Autodesk Inventor part; units mm, degrees
ref_plane "ip_cb_11_1_XY" through (2.3526, 9.0717, 3.7576) normal (1, 0, 0) x (0, 0, -1)
ref_plane "ip_cb_11_1_YZ" through (2.3526, 9.0717, 3.7576) normal (0, 0, -1) x (0, 1, 0)
ref_plane "ip_cb_11_1_ZX" through (2.3526, 9.0717, 3.7576) normal (0, 1, 0) x (1, 0, 0)
sketch "Sketch_1" plane through (0, 0, 0) normal (0, 0, 1) x (1, 0, 0)
  line L0 (14, 0) -> (0, 0)
  arc A0 (0, 5.6) -> (0.6, 5) centre (0.6, 5.6) ccw
  line L1 (0.6, 5) -> (13.4, 5)
  arc A1 (13.4, 5) -> (14, 5.6) centre (13.4, 5.6) ccw
  line L2 (14, 5.6) -> (14, 7.6)
  line L3 (14, 7.6) -> (12.4286, 7.6)
  arc A2 (10.8662, 7.6) -> (12.4286, 7.6) centre (11.6474, 9.8192) ccw
  line L4 (10.8662, 7.6) -> (3.1338, 7.6)
  arc A3 (1.5714, 7.6) -> (3.1338, 7.6) centre (2.3526, 9.8192) ccw
  line L5 (1.5714, 7.6) -> (0, 7.6)
  line L6 (0, 7.6) -> (0, 5.6)
revolve "Revolution1" add sketch "Sketch_1" angle 360 about axis through (14, 0, 0) along (1, 0, 0)
ref_plane "ip_cb_11_1_XY" through (2.3526, 9.0717, 3.7576) normal (1, 0, 0) x (0, 0, -1)
ref_plane "ip_cb_11_1_YZ" through (2.3526, 9.0717, 3.7576) normal (0, 0, -1) x (0, 1, 0)
ref_plane "ip_cb_11_1_ZX" through (2.3526, 9.0717, 3.7576) normal (0, 1, 0) x (1, 0, 0)
ref_plane "ip_cb_11_2_XY" through (2.3526, 3.7576, 9.0717) normal (1, 0, 0) x (0, 0, -1)
ref_plane "ip_cb_11_2_YZ" through (2.3526, 3.7576, 9.0717) normal (0, 0, -1) x (0, 1, 0)
ref_plane "ip_cb_11_2_ZX" through (2.3526, 3.7576, 9.0717) normal (0, 1, 0) x (1, 0, 0)
ref_plane "ip_cb_11_3_XY" through (2.3526, -3.7576, 9.0717) normal (1, 0, 0) x (0, 0, -1)
ref_plane "ip_cb_11_3_YZ" through (2.3526, -3.7576, 9.0717) normal (0, 0, -1) x (0, 1, 0)
ref_plane "ip_cb_11_3_ZX" through (2.3526, -3.7576, 9.0717) normal (0, 1, 0) x (1, 0, 0)
ref_plane "ip_cb_11_4_XY" through (2.3526, -9.0717, 3.7576) normal (1, 0, 0) x (0, 0, -1)
ref_plane "ip_cb_11_4_YZ" through (2.3526, -9.0717, 3.7576) normal (0, 0, -1) x (0, 1, 0)
ref_plane "ip_cb_11_4_ZX" through (2.3526, -9.0717, 3.7576) normal (0, 1, 0) x (1, 0, 0)
ref_plane "ip_cb_11_5_XY" through (2.3526, -9.0717, -3.7576) normal (1, 0, 0) x (0, 0, -1)
ref_plane "ip_cb_11_5_YZ" through (2.3526, -9.0717, -3.7576) normal (0, 0, -1) x (0, 1, 0)
ref_plane "ip_cb_11_5_ZX" through (2.3526, -9.0717, -3.7576) normal (0, 1, 0) x (1, 0, 0)
ref_plane "ip_cb_11_6_XY" through (2.3526, -3.7576, -9.0717) normal (1, 0, 0) x (0, 0, -1)
ref_plane "ip_cb_11_6_YZ" through (2.3526, -3.7576, -9.0717) normal (0, 0, -1) x (0, 1, 0)
ref_plane "ip_cb_11_6_ZX" through (2.3526, -3.7576, -9.0717) normal (0, 1, 0) x (1, 0, 0)
ref_plane "ip_cb_11_7_XY" through (2.3526, 3.7576, -9.0717) normal (1, 0, 0) x (0, 0, -1)
ref_plane "ip_cb_11_7_YZ" through (2.3526, 3.7576, -9.0717) normal (0, 0, -1) x (0, 1, 0)
ref_plane "ip_cb_11_7_ZX" through (2.3526, 3.7576, -9.0717) normal (0, 1, 0) x (1, 0, 0)
ref_plane "ip_cb_11_8_XY" through (2.3526, 9.0717, -3.7576) normal (1, 0, 0) x (0, 0, -1)
ref_plane "ip_cb_11_8_YZ" through (2.3526, 9.0717, -3.7576) normal (0, 0, -1) x (0, 1, 0)
ref_plane "ip_cb_11_8_ZX" through (2.3526, 9.0717, -3.7576) normal (0, 1, 0) x (1, 0, 0)
ref_plane "ip_cb_1a_XY" through (0, 0, 0) normal (-1, 0, 0) x (0, 0, -1)
ref_plane "ip_cb_1a_YZ" through (0, 0, 0) normal (0, 0, -1) x (0, -1, 0)
ref_plane "ip_cb_1a_ZX" through (0, 0, 0) normal (0, -1, 0) x (-1, 0, 0)
ref_plane "ip_cb_22_1_XY" through (11.6474, 9.8192, 0) normal (1, 0, 0) x (0, 0, -1)
ref_plane "ip_cb_22_1_YZ" through (11.6474, 9.8192, 0) normal (0, 0, -1) x (0, 1, 0)
ref_plane "ip_cb_22_1_ZX" through (11.6474, 9.8192, 0) normal (0, 1, 0) x (1, 0, 0)
ref_plane "ip_cb_22_2_XY" through (11.6474, 6.9432, 6.9432) normal (1, 0, 0) x (0, 0, -1)
ref_plane "ip_cb_22_2_YZ" through (11.6474, 6.9432, 6.9432) normal (0, 0, -1) x (0, 1, 0)
ref_plane "ip_cb_22_2_ZX" through (11.6474, 6.9432, 6.9432) normal (0, 1, 0) x (1, 0, 0)
ref_plane "ip_cb_22_3_XY" through (11.6474, 0, 9.8192) normal (1, 0, 0) x (0, 0, -1)
ref_plane "ip_cb_22_3_YZ" through (11.6474, 0, 9.8192) normal (0, 0, -1) x (0, 1, 0)
ref_plane "ip_cb_22_3_ZX" through (11.6474, 0, 9.8192) normal (0, 1, 0) x (1, 0, 0)
ref_plane "ip_cb_22_4_XY" through (11.6474, -6.9432, 6.9432) normal (1, 0, 0) x (0, 0, -1)
ref_plane "ip_cb_22_4_YZ" through (11.6474, -6.9432, 6.9432) normal (0, 0, -1) x (0, 1, 0)
ref_plane "ip_cb_22_4_ZX" through (11.6474, -6.9432, 6.9432) normal (0, 1, 0) x (1, 0, 0)
ref_plane "ip_cb_22_5_XY" through (11.6474, -9.8192, 0) normal (1, 0, 0) x (0, 0, -1)
ref_plane "ip_cb_22_5_YZ" through (11.6474, -9.8192, 0) normal (0, 0, -1) x (0, 1, 0)
ref_plane "ip_cb_22_5_ZX" through (11.6474, -9.8192, 0) normal (0, 1, 0) x (1, 0, 0)
ref_plane "ip_cb_22_6_XY" through (11.6474, -6.9432, -6.9432) normal (1, 0, 0) x (0, 0, -1)
ref_plane "ip_cb_22_6_YZ" through (11.6474, -6.9432, -6.9432) normal (0, 0, -1) x (0, 1, 0)
ref_plane "ip_cb_22_6_ZX" through (11.6474, -6.9432, -6.9432) normal (0, 1, 0) x (1, 0, 0)
ref_plane "ip_cb_22_7_XY" through (11.6474, 0, -9.8192) normal (1, 0, 0) x (0, 0, -1)
ref_plane "ip_cb_22_7_YZ" through (11.6474, 0, -9.8192) normal (0, 0, -1) x (0, 1, 0)
ref_plane "ip_cb_22_7_ZX" through (11.6474, 0, -9.8192) normal (0, 1, 0) x (1, 0, 0)
ref_plane "ip_cb_22_8_XY" through (11.6474, 6.9432, -6.9432) normal (1, 0, 0) x (0, 0, -1)
ref_plane "ip_cb_22_8_YZ" through (11.6474, 6.9432, -6.9432) normal (0, 0, -1) x (0, 1, 0)
ref_plane "ip_cb_22_8_ZX" through (11.6474, 6.9432, -6.9432) normal (0, 1, 0) x (1, 0, 0)
properties part number "2200 Inner Ring"
The model under review builds one solid part; all positions refer to its coordinate system, in mm. Round coordinates to 2 decimals unless told otherwise and drop trailing zeros. Order: outer loops, then holes, each group sorted by start corner. A loop starts at its lowest first (then second) coordinate and runs counter-clockwise, first axis right, second up. Notation, with made-up numbers: (30, -10) -> (88, -10) arc R14 ccw to (88, 9) -> close; hole circle Ø10 at (-27, -32.75). An arc over 180 degrees is marked (long way). Use a Markdown table: item, result.
Q1. Clearance check with flat-ended pins moving along their axes: P1, Ø1.5, axis at x = 3.5, y = 2.5, coming from the +Z side; P2, Ø1, axis at x = 7, z = 2, coming from the +Y side; P3, Ø1.5, axis at x = 12, z = -5.5, coming from the -Y side. State where each tip first meets the part, or that it passes through.
Values:
| item | result |
|---|---|
| P1 | stops at z = 7.4 |
| P2 | stops at y = 7.45 |
| P3 | stops at y = -5.83 |
Q2. We need section C-C on x = 10. Write out the cut boundary in (y, z), then the cut area to 3 significant figures.
Values:
| item | result |
|---|---|
| outline | circle Ø15.2 at (0, 0); hole circle Ø10 at (0, 0) |
| area | 103 mm^2 |
Q3. For line 1 (Z direction, x = 4, y = 0); line 2 (Z direction, x = 11.25, y = 0.75); line 3 (Y direction, x = 9.75, z = 2.25), list the stretches that pass through material, from the lowest coordinate up.
Values:
| item | result |
|---|---|
| line 1 | z = -7.6 to -5, 5 to 7.6 |
| line 2 | z = -7.46 to -4.94, 4.94 to 7.46 |
| line 3 | y = -7.26 to -4.47, 4.47 to 7.26 |
Q4. Mouldability with a two-part tool opening along Z and no side actions: class faces 1 (the flat face through (0, -1, -6)), 2 (the cylindrical face through (6.946, -7.593, -0.334)), 3 (the cylindrical face through (7.09, -1.08, -4.88)) as +Z half, -Z half, draft (parallel to the pull), parting line (faces both ways), or undercut.
Values:
| item | result |
|---|---|
| face 1 | draft |
| face 2 | parting line |
| face 3 | undercut |
Q5. We need section A-A on z = 0. Write out the cut boundary in (x, y), then the cut area to 3 significant figures.
Values:
| item | result |
|---|---|
| outline | (0, -7.6) -> (1.57, -7.6) arc R2.35 cw to (3.13, -7.6) -> (10.87, -7.6) arc R2.35 cw to (12.43, -7.6) -> (14, -7.6) -> (14, -5.6) arc R0.6 ccw to (13.4, -5) -> (0.6, -5) arc R0.6 ccw to (0, -5.6) -> close; (0, 5.6) arc R0.6 ccw to (0.6, 5) -> (13.4, 5) arc R0.6 ccw to (14, 5.6) -> (14, 7.6) -> (12.43, 7.6) arc R2.35 cw to (10.87, 7.6) -> (3.13, 7.6) arc R2.35 cw to (1.57, 7.6) -> (0, 7.6) -> close |
| area | 71.9 mm^2 |
